Source: three-view drawing plus pictorial views. Frame: mm from the lowest corner of the part. A direction names the side the tool comes from. Give positions to 0.01 mm unless a question says otherwise; leave off trailing zeros. Order: outer loops, then holes, each group sorted by start corner. A loop starts at its lowest first (then second) coordinate and runs counter-clockwise, first axis right, second up. Notation, with made-up numbers: (68.25, 71) -> (93.25, 71) arc R3 ccw to (93.25, 76) -> close; hole circle Ø8 at (21, 13). An arc over 180 degrees is marked (long way). Use a Markdown table: item, result. Add a question column.
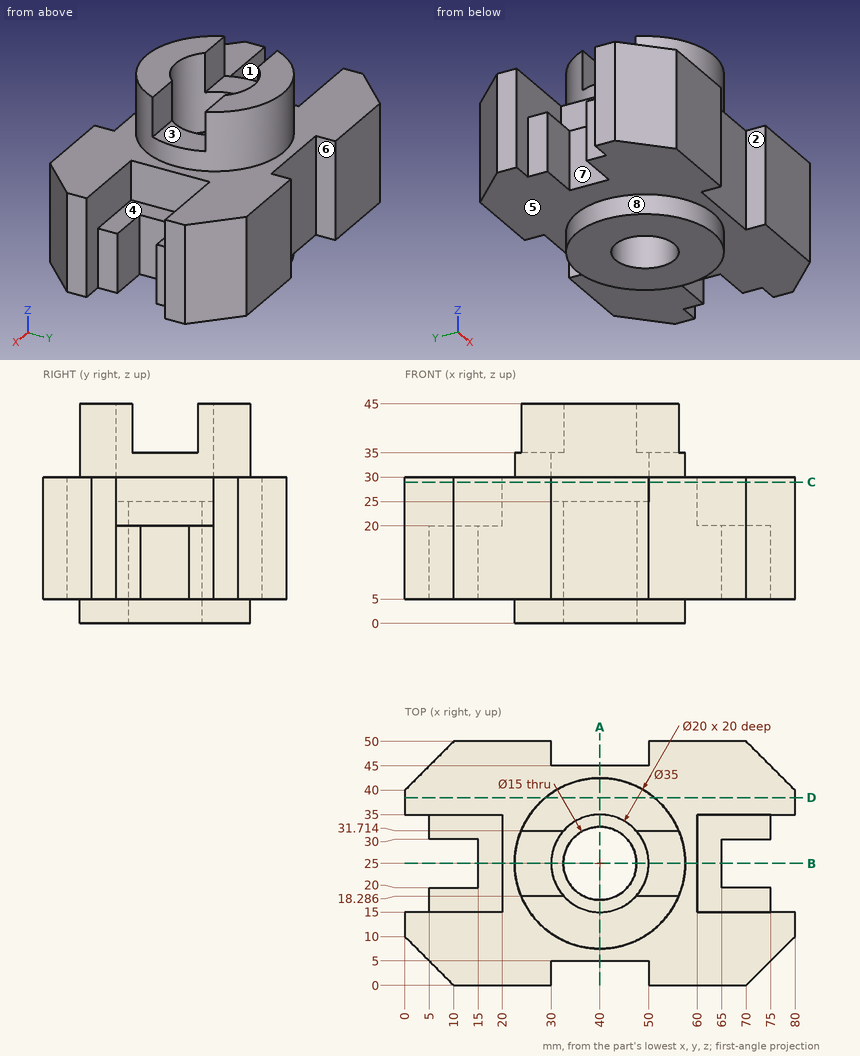
Q1. Section query C-C (z = 29). Return loops of the section in (x, y), plus the area to 3 significant figures.
Q2. Section query A-A (x = 40). Return loops of the section in (y, z).
Q3. Ray query, line 1 (Y direction, x = 40, z = 11); line 2 (X direction, y = 25, z = 24.5); line 3 (X direction, y = 25, z = 16). Return the intervals inside material, ascending.
Q4. Access query for the marked faces 1, 2, 3, 4 and 5. Directions: +Z, -Z, +X, -X, +Y, -Y. A direction counts if a zero-diameter tool reaches every point of the face in a straight line with its end or side. Return the directions, or none.
Q5. Draft query along Y for the marked faces 6, 7 and 8. Return one class per face: +Y half, -Y half, draft (parallel to the pull), parting line (faces both ways), or undercut.
Q6. First-contact query: pin 1 (5.5 mm diameter, centred on y = 2.5, z = 13.5, fed in from -X); pin 2 (6 mm diameter, centred on x = 16, y = 15.5, fed in from +Z); pin 3 (1 mm diameter, centred on y = 27.5, z = 6.5, fed in from -X). Flat tips, straight axial feed; report the tip coordinate or a pass-through.
Q7. Section query D-D (y = 38.5). Return loops of the section in (x, z) (1 decimal).
Q8. Section query B-B (y = 25). Return loops of the section in (x, z).
Solution:
| question | item | result |
|---|---|---|
| 1 | outline | (0, 10) -> (10, 0) -> (30, 0) -> (30, 5) -> (50, 5) -> (50, 0) -> (70, 0) -> (80, 10) -> (80, 15) -> (60, 15) -> (60, 35) -> (80, 35) -> (80, 40) -> (70, 50) -> (50, 50) -> (50, 45) -> (30, 45) -> (30, 50) -> (10, 50) -> (0, 40) -> (0, 35) -> (20, 35) -> (20, 15) -> (0, 15) -> close; hole circle Ø20 at (40, 25) |
| 1 | area | 2,490 mm² |
| 2 | outline | (5, 5) -> (7.5, 5) -> (7.5, 0) -> (17.5, 0) -> (17.5, 25) -> (15, 25) -> (15, 45) -> (7.5, 45) -> (7.5, 30) -> (5, 30) -> close; (32.5, 0) -> (42.5, 0) -> (42.5, 5) -> (45, 5) -> (45, 30) -> (42.5, 30) -> (42.5, 45) -> (35, 45) -> (35, 25) -> (32.5, 25) -> close |
| 3 | line 1 | y = 5 to 17.5, 32.5 to 45 |
| 3 | line 2 | x = 20 to 32.5, 47.5 to 60 |
| 3 | line 3 | x = 15 to 32.5, 47.5 to 65 |
| 4 | face 1 | +Z, -X |
| 4 | face 2 | +Z, -Z, -Y |
| 4 | face 3 | +Z, +X, -X |
| 4 | face 4 | +Z, +X |
| 4 | face 5 | -Z |
| 5 | face 6 | draft |
| 5 | face 7 | undercut |
| 5 | face 8 | parting line |
| 6 | pin 1 | stops at x = 4.75 |
| 6 | pin 2 | stops at z = 30 |
| 6 | pin 3 | stops at x = 15 |
| 7 | outline | (0, 5) -> (28.9, 5) -> (28.9, 0) -> (51.1, 0) -> (51.1, 5) -> (80, 5) -> (80, 30) -> (51.1, 30) -> (51.1, 45) -> (28.9, 45) -> (28.9, 30) -> (0, 30) -> close |
| 8 | outline | (15, 5) -> (22.5, 5) -> (22.5, 0) -> (32.5, 0) -> (32.5, 25) -> (30, 25) -> (30, 35) -> (22.5, 35) -> (22.5, 30) -> (20, 30) -> (20, 20) -> (15, 20) -> close; (47.5, 0) -> (57.5, 0) -> (57.5, 5) -> (65, 5) -> (65, 20) -> (60, 20) -> (60, 30) -> (57.5, 30) -> (57.5, 35) -> (50, 35) -> (50, 25) -> (47.5, 25) -> close |
